Source: CAD feature listing. Evaluate the final solid. Frame: model axes, mm. Give positions to 0.01 mm unless a question says otherwise; leave off trailing zeros. Loops run counter-clockwise (first coordinate to the right, second up) from the corner with the lowest first, then second, coordinate; pieces in that order, holes last. Notation, with made-up numbers: M 72.5,24.25 L 102.5,24.25 A21 ccw 102.5,53.25 Z; hole C -9,46.25 d7. An arc over 180 degrees is marked long. Write item = value, one per line.
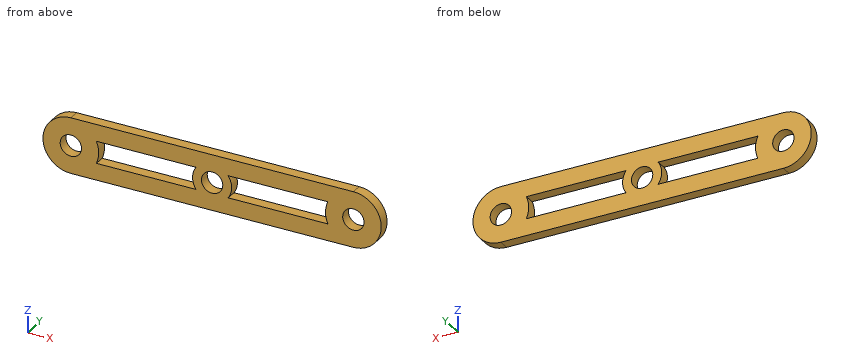
from build123d import *

# Parameters (mm, degrees)
SKETCH1_R           = 1.5875
BOSS_EXTRUDE2_DEPTH = 0.79375


with BuildPart() as part:
    # Sketch1 → Boss-Extrude2 (new, symmetric)
    with BuildSketch(Plane(origin=(0, 0, 0), x_dir=(1, 0, 0), z_dir=(0, 1, 0))):
        with BuildLine():
            Line((21, 4.15), (-21, 4.15))
            ThreePointArc((-21, 4.15), (-25.15, 0), (-21, -4.15))
            Line((-21, -4.15), (21, -4.15))
            ThreePointArc((21, -4.15), (25.15, 0), (21, 4.15))
        make_face()
        with Locations(Location((21, 0, 0), (0, 0, 270))):
            Circle(SKETCH1_R, mode=Mode.SUBTRACT)
        with Locations(Location((-21, 0, 0), (0, 0, 270))):
            Circle(SKETCH1_R, mode=Mode.SUBTRACT)
        with Locations(Location((0, 0, 0), (0, 0, 270))):
            Circle(SKETCH1_R, mode=Mode.SUBTRACT)
        with BuildLine():
            Line((17.202806092, 1.65), (2.390587638, 1.65))
            ThreePointArc((2.390587638, 1.65), (2.904721889, 0), (2.390587638, -1.65))
            Line((2.390587638, -1.65), (17.202806092, -1.65))
            ThreePointArc((17.202806092, -1.65), (16.859808992, 0), (17.202806092, 1.65))
        make_face(mode=Mode.SUBTRACT)
        with BuildLine():
            Line((-17.202806092, -1.65), (-2.390587638, -1.65))
            ThreePointArc((-2.390587638, -1.65), (-2.904721889, 0), (-2.390587638, 1.65))
            Line((-2.390587638, 1.65), (-17.202806092, 1.65))
            ThreePointArc((-17.202806092, 1.65), (-16.859808992, 0), (-17.202806092, -1.65))
        make_face(mode=Mode.SUBTRACT)
    extrude(amount=BOSS_EXTRUDE2_DEPTH, both=True)


solid = part.part
1. Cut plane B-B, the plane x = 5. Return the cut outline in (y, z), then the cut area to 3 significant figures.
Derived:
outline = M -0.79,-4.15 L 0.79,-4.15 L 0.79,-1.65 L -0.79,-1.65 Z; M -0.79,1.65 L 0.79,1.65 L 0.79,4.15 L -0.79,4.15 Z
area = 7.94 mm²
2. Cut plane D-D, the plane z = -3. Return the cut outline in (x, y).
Derived:
outline = M -23.87,-0.79 L 23.87,-0.79 L 23.87,0.79 L -23.87,0.79 Z
3. Cut plane C-C, the plane y = -0.3. Count the separate pieces of the cut face and the enclosed holes in it, then the cut area to 3 significant figures.
Derived:
separate_pieces = 1
enclosed_holes = 5
area = 285 mm²
4. Cut plane A-A, the plane z = 0. Return the cut outline in (x, y).
Derived:
outline = M -25.15,-0.79 L -22.59,-0.79 L -22.59,0.79 L -25.15,0.79 Z; M -19.41,-0.79 L -16.86,-0.79 L -16.86,0.79 L -19.41,0.79 Z; M -2.9,-0.79 L -1.59,-0.79 L -1.59,0.79 L -2.9,0.79 Z; M 1.59,-0.79 L 2.9,-0.79 L 2.9,0.79 L 1.59,0.79 Z; M 16.86,-0.79 L 19.41,-0.79 L 19.41,0.79 L 16.86,0.79 Z; M 22.59,-0.79 L 25.15,-0.79 L 25.15,0.79 L 22.59,0.79 Z
5. Material intervals for probe 1 along Z at (x, y) = (12.5, -0.05); probe 2 along X at (y, z) = (-0.65, -0.25); probe 3 along Z at (x, y) = (20.5, 0.55), sorted ascending. Write a range as from..to.
Derived:
probe_1 = -4.15..-1.65, 1.65..4.15
probe_2 = -25.14..-22.57, -19.43..-16.87, -2.89..-1.57, 1.57..2.89, 16.87..19.43, 22.57..25.14
probe_3 = -4.15..-1.51, 1.51..4.15
